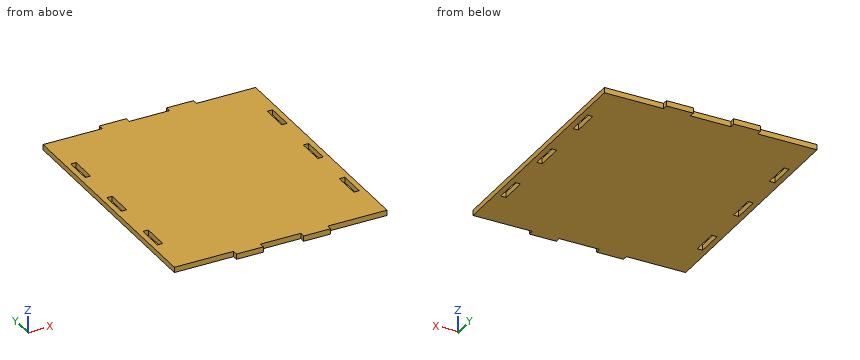
Solid Edge part; units mm, degrees
sketch "Sketch1" plane through (0, 0, 0) normal (0, 0, 1) x (1, 0, 0)
  line L0 (7.5, -60.5) -> (-7.5, -60.5)
  line L1 (-7.5, -60.5) -> (-7.5, -62.5)
  line L2 (-7.5, -62.5) -> (-17.5, -62.5)
  line L3 (-17.5, -62.5) -> (-17.5, -60.5)
  line L4 (-17.5, -60.5) -> (-39.5, -60.5)
  line L5 (-39.5, -60.5) -> (-39.5, 30.5)
  line L6 (-39.5, 30.5) -> (-17.5, 30.5)
  line L7 (-17.5, 30.5) -> (-17.5, 32.5)
  line L8 (-17.5, 32.5) -> (-7.5, 32.5)
  line L9 (-7.5, 32.5) -> (-7.5, 30.5)
  line L10 (-7.5, 30.5) -> (7.5, 30.5)
  line L11 (7.5, 30.5) -> (7.5, 32.5)
  line L12 (7.5, 32.5) -> (17.5, 32.5)
  line L13 (17.5, 32.5) -> (17.5, 30.5)
  line L14 (17.5, 30.5) -> (39.5, 30.5)
  line L15 (39.5, 30.5) -> (39.5, -60.5)
  line L16 (39.5, -60.5) -> (17.5, -60.5)
  line L17 (17.5, -60.5) -> (17.5, -62.5)
  line L18 (17.5, -62.5) -> (7.5, -62.5)
  line L19 (7.5, -62.5) -> (7.5, -60.5)
  line L20 (37.5, 5) -> (37.5, 15)
  line L21 (35.5, 5) -> (37.5, 5)
  line L22 (35.5, 15) -> (35.5, 5)
  line L23 (37.5, 15) -> (35.5, 15)
  line L24 (-35.5, -45) -> (-35.5, -35)
  line L25 (-37.5, -45) -> (-35.5, -45)
  line L26 (-37.5, -35) -> (-37.5, -45)
  line L27 (-35.5, -35) -> (-37.5, -35)
  line L28 (-37.5, 15) -> (-37.5, 5)
  line L29 (-35.5, 15) -> (-37.5, 15)
  line L30 (-35.5, 5) -> (-35.5, 15)
  line L31 (-37.5, 5) -> (-35.5, 5)
  line L32 (35.5, -45) -> (37.5, -45)
  line L33 (35.5, -35) -> (35.5, -45)
  line L34 (37.5, -35) -> (35.5, -35)
  line L35 (37.5, -45) -> (37.5, -35)
  line L36 (37.5, -20) -> (37.5, -10)
  line L37 (35.5, -20) -> (37.5, -20)
  line L38 (35.5, -10) -> (35.5, -20)
  line L39 (37.5, -10) -> (35.5, -10)
  line L40 (-37.5, -20) -> (-35.5, -20)
  line L41 (-37.5, -10) -> (-37.5, -20)
  line L42 (-35.5, -10) -> (-37.5, -10)
  line L43 (-35.5, -20) -> (-35.5, -10)
extrude "Protrusion1" add sketch "Sketch1" along normal blind 2
properties material "Acrylic, high impact grade"
Work out the finished part from the listing and answer in its coordinate system (mm). Give positions to 0.01 mm unless a question says otherwise; leave off trailing zeros. Loops run counter-clockwise (first coordinate to the right, second up) from the corner with the lowest first, then second, coordinate; pieces in that order, holes last. Notation, with made-up numbers: (82.5, 18) -> (131.5, 18) arc R34 ccw to (131.5, 56) -> close; hole circle Ø1 at (54.5, 39). An arc over 180 degrees is marked (long way). Write item = value, one per line. Start each with the question number.
(1) Find section B-B on x = 2.5. Give the vertices of the cut face in (y, z).
(2) Find section C-C on z = 1. Give the number of separate pieces and of enclosed holes in the cut face, and give its area (3 significant figures).
(3) Given pin 1 Ø1 at (x, z) = (-37, 1.5) entering from -Y; pin 2 Ø0.6 at (x, z) = (36.5, 0.5) entering from +Y; pin 3 Ø1 at (y, z) = (31.5, 1.5) entering from +X, each flat-ended and moving along its own axis, determine where each tip first touches the part or whether it passes through.
(4) Find the intervals of material crossed by probe 1 along X at (y, z) = (14.5, 1.65); probe 2 along Y at (x, z) = (-31.5, 0.45), in increasing order. Write a range as from..to.
(5) Find section A-A on y = 14. Give the vertices of the cut face in (x, z), and give its area (3 significant figures).
From the geometry:
q1.outline = (-60.5, 0) -> (30.5, 0) -> (30.5, 2) -> (-60.5, 2) -> close
q2.separate_pieces = 1
q2.enclosed_holes = 6
q2.area = 7,150 mm^2
q3.pin_1 = -60.5
q3.pin_2 = 30.5
q3.pin_3 = 17.5
q4.probe_1 = -39.5..-37.5, -35.5..35.5, 37.5..39.5
q4.probe_2 = -60.5..30.5
q5.outline = (-39.5, 0) -> (-37.5, 0) -> (-37.5, 2) -> (-39.5, 2) -> close; (-35.5, 0) -> (35.5, 0) -> (35.5, 2) -> (-35.5, 2) -> close; (37.5, 0) -> (39.5, 0) -> (39.5, 2) -> (37.5, 2) -> close
q5.area = 150 mm^2
